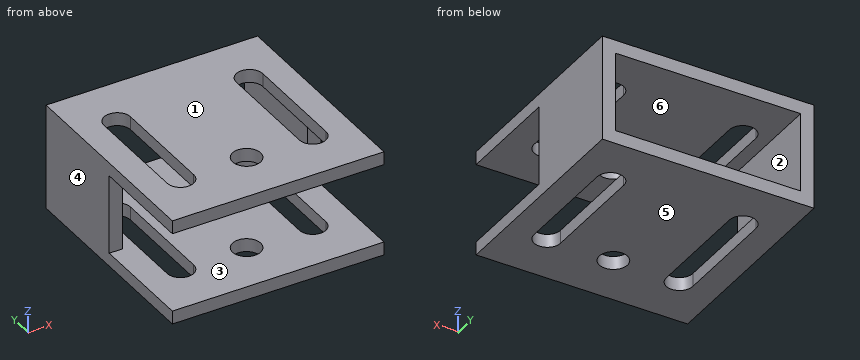
Autodesk Inventor part; units mm, degrees
ref_plane "YZ Plane" through (0, 0, 0) normal (1, 0, 0) x (0, 1, 0)
ref_plane "XZ Plane" through (0, 0, 0) normal (0, 1, 0) x (-1, 0, 0)
ref_plane "XY Plane" through (0, 0, 0) normal (0, 0, 1) x (1, 0, 0)
ref_plane "Work Plane1" through (0, 50.8, 0) normal (0, 1, 0) x (0, 0, -1)
sketch "Sketch1" plane through (0, 50.8, 0) normal (0, 1, 0) x (0, 0, -1)
  line L0 (0, 50.8) -> (-25.4, 50.8)
  line L1 (-25.4, 50.8) -> (-25.4, 0)
  line L2 (-25.4, 0) -> (0, 0)
  line L3 (0, 0) -> (0, 50.8)
  line L4 (-3.175, 3.175) -> (-22.225, 3.175)
  line L5 (-22.225, 3.175) -> (-22.225, 47.625)
  line L6 (-22.225, 47.625) -> (-3.175, 47.625)
  line L7 (-3.175, 47.625) -> (-3.175, 3.175)
  point P0 (0, 0)
  dimension "d0" = 25.4
  dimension "d1" = 50.8
  dimension "d9" = 3.175
extrude "Extrusion3" add sketch "Sketch1" along normal blind 50.8
sketch "Sketch3" plane through (-50.8, 50.8, 25.4) normal (0, 0, 1) x (1, 0, 0)
  circle A0 centre (25.4, 12.7) radius 3.3734
  line L0 (0, 0) -> (50.8, 0)
  line L1 (0, 0) -> (0, 50.8)
  line L2 (41.275, 38.1) -> (41.275, 12.7) construction
  line L3 (38.1, 38.1) -> (38.1, 12.7)
  line L4 (44.45, 12.7) -> (44.45, 38.1)
  arc A1 (44.45, 38.1) -> (38.1, 38.1) centre (41.275, 38.1) ccw
  arc A2 (38.1, 12.7) -> (44.45, 12.7) centre (41.275, 12.7) ccw
  line L5 (50.8, 0) -> (50.8, 50.8)
  line L6 (3.175, 0) -> (47.625, 0) construction
  line L7 (25.4, 0) -> (25.4, 50.8) construction
  line L8 (47.625, 50.8) -> (3.175, 50.8) construction
  line L9 (12.7, 38.1) -> (12.7, 12.7)
  line L10 (6.35, 12.7) -> (6.35, 38.1)
  arc A3 (12.7, 38.1) -> (6.35, 38.1) centre (9.525, 38.1) ccw
  arc A4 (6.35, 12.7) -> (12.7, 12.7) centre (9.525, 12.7) ccw
  point P0 (50.8, -50.8)
  point P1 (41.275, 25.4)
  dimension "d12" = 6.7469
  dimension "d13" = 12.7
  dimension "d14" = 25.4
  dimension "d20" = 6.35
  dimension "d21" = 25.4
  dimension "d22" = 9.525
  dimension "d23" = 25.4
extrude "Extrusion4" cut sketch "Sketch3" against normal blind 25.4
sketch "Sketch4" plane through (0, 50.8, 25.4) normal (1, 0, 0) x (0, 0, -1)
  line L0 (3.175, 0) -> (3.175, 50.8)
  line L1 (22.225, 0) -> (22.225, 50.8)
  line L2 (3.175, 0) -> (22.225, 0)
  line L3 (22.225, 0) -> (22.225, 25.4)
  line L4 (22.225, 25.4) -> (3.175, 25.4)
  line L5 (3.175, 25.4) -> (3.175, 0)
  point P0 (25.4, -50.8)
  dimension "d17" = 25.4
extrude "Extrusion5" cut sketch "Sketch4" against normal blind 50.8
properties part number "block"
Input: part model. Units: mm. Frame: model coordinates. Face numbers are marked on the shaded views. A direction names the side the tool comes from. Coordinates: 2 decimals unless noted, no trailing zeros. Loops run counter-clockwise (first coordinate to the right, second up) from the corner with the lowest first, then second, coordinate; pieces in that order, holes last. Notation, with made-up numbers: (-24, 87) -> (22, 87) arc R17 ccw to (22, 96) -> close; hole circle Ø1 at (2.25, 28.25). An arc over 180 degrees is marked (long way). Write item = value, one per line. Start each with the question number.
Item 1: Reachability of the marked faces 1 and 2 from +Z, -Z, +X, -X, +Y, -Y: full face, straight path, thin tool, end or side. Return the list, or none.
Item 2: Cut plane B-B, the plane x = -16. Return loops of the section in (y, z) (3 decimals), plus the area to 3 significant figures.
Item 3: Cut plane C-C, the plane z = 4.75. Return loops of the section in (x, y) (3 decimals), plus the area to 3 significant figures.
Item 4: Mould query, pull axis Z, two halves, no side actions, for the marked faces 3, 4, 5 and 6. Classes: pulls with the +Z half, pulls with the -Z half, needs draft (parallel to the pull), parting line crosses it, or undercut.
Item 5: Cut plane D-D, the plane x = -25.4. Return loops of the section in (y, z) (3 decimals), plus the area to 3 significant figures.
Item 6: Cut plane A-A, the plane y = 88. Return loops of the section in (x, z) (3 decimals).
Item 7: First-contact query: P1, Ø8, axis at x = -12.5, z = 14.5, coming from the -Y side; P2, Ø1.6, axis at x = -49, z = 16, coming from the -Y side. Flat tips, straight axial feed; report the tip coordinate or a pass-through.
Item 8: Material intervals for line 1 (Z direction, x = -27, y = 73.5) (3 decimals); line 2 (X direction, y = 78, z = 18.5) (3 decimals); line 3 (Y direction, x = -25.4, z = 1.4), sorted ascending.
Ans:
q1.face_1 = +Z, +X, -X, +Y, -Y
q1.face_2 = +Y, -Y
q2.outline = (50.8, 0) -> (101.6, 0) -> (101.6, 3.175) -> (50.8, 3.175) -> close; (50.8, 22.225) -> (101.6, 22.225) -> (101.6, 25.4) -> (50.8, 25.4) -> close
q2.area = 323 mm²
q3.outline = (-50.8, 76.2) -> (-47.625, 76.2) -> (-47.625, 101.6) -> (-50.8, 101.6) -> close; (-3.175, 76.2) -> (0, 76.2) -> (0, 101.6) -> (-3.175, 101.6) -> close
q3.area = 161 mm²
q4.face_3 = undercut
q4.face_4 = needs draft
q4.face_5 = pulls with the -Z half
q4.face_6 = undercut
q5.outline = (50.8, 0) -> (60.127, 0) -> (60.127, 3.175) -> (50.8, 3.175) -> close; (50.8, 22.225) -> (60.127, 22.225) -> (60.127, 25.4) -> (50.8, 25.4) -> close; (66.873, 0) -> (101.6, 0) -> (101.6, 3.175) -> (66.873, 3.175) -> close; (66.873, 22.225) -> (101.6, 22.225) -> (101.6, 25.4) -> (66.873, 25.4) -> close
q5.area = 280 mm²
q6.outline = (-50.8, 0) -> (-44.45, 0) -> (-44.45, 3.175) -> (-47.625, 3.175) -> (-47.625, 22.225) -> (-44.45, 22.225) -> (-44.45, 25.4) -> (-50.8, 25.4) -> close; (-38.1, 0) -> (-12.7, 0) -> (-12.7, 3.175) -> (-38.1, 3.175) -> close; (-38.1, 22.225) -> (-12.7, 22.225) -> (-12.7, 25.4) -> (-38.1, 25.4) -> close; (-6.35, 0) -> (0, 0) -> (0, 25.4) -> (-6.35, 25.4) -> (-6.35, 22.225) -> (-3.175, 22.225) -> (-3.175, 3.175) -> (-6.35, 3.175) -> close
q7.P1 = through
q7.P2 = 76.2
q8.line_1 = 0 to 3.175, 22.225 to 25.4
q8.line_2 = -50.8 to -47.625, -3.175 to 0
q8.line_3 = 50.8 to 60.13, 66.87 to 101.6
